Geometry: final body of the model. Coordinates: model frame, mm. A direction names the side the tool comes from. Give positions to 0.01 mm unless a question says otherwise; leave off trailing zeros.
from build123d import *

# Parameters (mm, degrees)
ESBO_O1_W                = 192
ESBO_O1_H                = 50
RESSALTO_EXTRUS_O1_DEPTH = 6
ESBO_O2_R                = 1.5
CORTE_EXTRUS_O1_DEPTH    = 15


with BuildPart() as part:
    # Esboço1 → Ressalto-extrusão1 (new, symmetric)
    with BuildSketch(Plane.XY):
        Rectangle(ESBO_O1_W, ESBO_O1_H)
    extrude(amount=RESSALTO_EXTRUS_O1_DEPTH, both=True)

    # Esboço2 → Corte-extrusão1 (cut, symmetric)
    with BuildSketch(Plane(origin=(0, -25, 0), x_dir=(-1, 0, 0), z_dir=(0, -1, 0))):
        with Locations(Location((77.5, 0, 0), (0, 0, 90))):
            Circle(ESBO_O2_R)
        with Locations(Location((-77.5, 0, 0), (0, 0, 90))):
            Circle(ESBO_O2_R)
    extrude(amount=CORTE_EXTRUS_O1_DEPTH, both=True, mode=Mode.SUBTRACT)


solid = part.part
Q1. Pull-direction query (Z, two-part tool) for faces 1 (the flat face through (-1, 25, 0)), 2 (the flat face through (-1, 0, 6)), 3 (the cylindrical face through (-76.235, -17.605, -0.806)); classes: released by +Z, released by -Z, zero draft, split by the parting line, or undercut.
Filled sheet:
face 1: zero draft
face 2: released by +Z
face 3: undercut
Q2. Pin query (flat end, axial travel): P1, Ø2.5, axis at x = -77.5, z = 0, coming from the -Y side; P2, Ø3.5, axis at x = -77, z = 0.5, coming from the -Y side. Return the tip coordinate at first contact, or that it passes through.
Filled sheet:
P1: stops at y = -10
P2: stops at y = -25
Q3. Ray query, line 1 along X through (y, z) = (-19.5, 0); line 2 along Z through (x, y) = (77.5, -14); line 3 along Z through (x, y) = (77, -20). Return the intervals inside material, ascending.
Filled sheet:
line 1: x = -96 to -79, -76 to 76, 79 to 96
line 2: z = -6 to -1.5, 1.5 to 6
line 3: z = -6 to -1.41, 1.41 to 6
Q4. Access query for faces 4 (the flat face through (-1, -25, 0)), 5 (the flat face through (-77, -10, 0)). Directions: +Z, -Z, +X, -X, +Y, -Y. A direction counts if a zero-diameter tool reaches every point of the face in a straight line with its end or side. Return the directions, or none.
Filled sheet:
face 4: +Z, -Z, +X, -X, -Y
face 5: -Y
